Here's how the part is built. I have some questions about the finished solid (model axes, mm). Face numbers are marked on the shaded views. Round coordinates to 2 decimals unless told otherwise and drop trailing zeros. Order: outer loops, then holes, each group sorted by start corner. A loop starts at its lowest first (then second) coordinate and runs counter-clockwise, first axis right, second up. Notation, with made-up numbers: (25.25, 86.25) -> (58.25, 86.25) arc R29 ccw to (58.25, 106.25) -> close; hole circle Ø4 at (82.25, -4). An arc over 180 degrees is marked (long way). One line per item, written item: value.
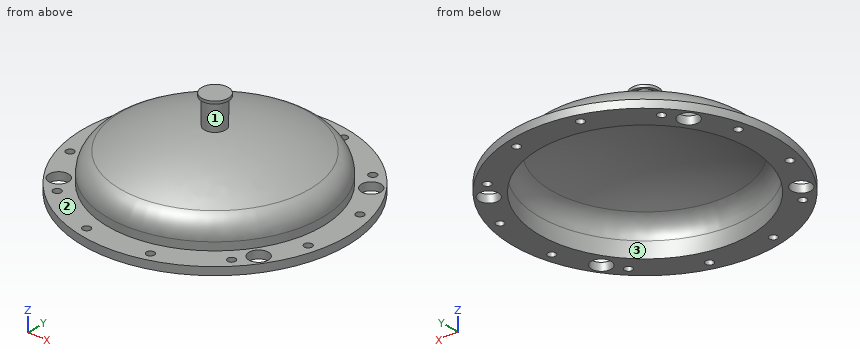
```python
from build123d import *

# Parameters (mm, degrees)
F2_R          = 250
F2_R_2        = 200
F3_DEPTH      = 10
F3_DEPTH_BACK = 5
F4_R          = 7.5
F5_DEPTH      = 15
F7_R          = 20
F9_R          = 25.25
F10_DEPTH     = 5
F11_R         = 18.5
F12_DEPTH     = 20


with BuildPart() as f1:
    # F0 (on Front) → F1 (revolve)
    with BuildSketch(Plane.XZ):
        with BuildLine():
            Line((200, 20), (200, 0))
            Line((200, 0), (203, 0))
            Line((203, 0), (203, 20))
            ThreePointArc((203, 20), (196.5493669363, 42.6526770285), (179.1328476019, 58.5088839444))
            ThreePointArc((179.1328476019, 58.5088839444), (92.0009441475, 89.9153591058), (0, 100.6000003082))
            Line((0, 100.6000003082), (0, 97.6))
            ThreePointArc((0, 97.6), (91.3153782925, 86.994742746), (177.7979977692, 55.8222176227))
            ThreePointArc((177.7979977692, 55.8222176227), (193.9994111035, 41.072257701), (200, 20))
        make_face()
    revolve(axis=Axis((0, 0, 99.1000001541), (0, 0, 1)))

    # F2 (on face) → F3 (join, two sides)
    with BuildSketch(Plane(origin=(0, 0, 0), x_dir=(1, 0, 0), z_dir=(0, 0, -1))) as f3_sk:
        Circle(F2_R)
        Circle(F2_R_2, mode=Mode.SUBTRACT)
    extrude(amount=F3_DEPTH)
    extrude(f3_sk.sketch, amount=-F3_DEPTH_BACK)

    # F4 (on face) → F5 (cut, through all)
    with BuildSketch(Plane.XY.offset(5)):
        with Locations((222.8771156759, 58.8813327608)):
            Circle(F4_R)
        with Locations((163.5765777171, 162.4312878175)):
            Circle(F4_R)
        with Locations((60.4458278584, 222.457910478)):
            Circle(F4_R)
        with Locations((-58.8813327608, 222.8771156759)):
            Circle(F4_R)
        with Locations((-162.4312878175, 163.5765777171)):
            Circle(F4_R)
        with Locations((-222.457910478, 60.4458278584)):
            Circle(F4_R)
        with Locations((-222.8771156759, -58.8813327608)):
            Circle(F4_R)
        with Locations((-163.5765777171, -162.4312878175)):
            Circle(F4_R)
        with Locations((-60.4458278584, -222.457910478)):
            Circle(F4_R)
        with Locations((58.8813327608, -222.8771156759)):
            Circle(F4_R)
        with Locations((162.4312878175, -163.5765777171)):
            Circle(F4_R)
        with Locations((222.457910478, -60.4458278584)):
            Circle(F4_R)
    extrude(amount=-F5_DEPTH, mode=Mode.SUBTRACT)

    # F7 (on offset) → F8 (join, up to the next surface of F1)
    with BuildSketch(Plane.XY.offset(150)):
        Circle(F7_R)
    extrude(until=Until.NEXT, dir=(0, 0, -1))

    # F9 (on face) → F10 (join)
    with BuildSketch(Plane.XY.offset(150)):
        Circle(F9_R)
    extrude(amount=F10_DEPTH)

    # F11 (on face) → F12 (cut)
    with BuildSketch(Plane.XY.offset(5)):
        with Locations((186.3570900757, 130.4886392699)):
            Circle(F11_R)
        with Locations((-186.3570900757, 130.4886392699)):
            Circle(F11_R)
        with Locations((-186.3570900757, -130.4886392699)):
            Circle(F11_R)
        with Locations((186.3570900757, -130.4886392699)):
            Circle(F11_R)
    extrude(amount=-F12_DEPTH, mode=Mode.SUBTRACT)


solid = f1.part
```
Q1. If we mould it in two halves opening along X, with no side actions, what happens to the marked faces 1, 2 and 3? For each: pulls with the +X half, pulls with the -X half, needs draft (parallel to the pull), parting line crosses it, or undercut.
Answers:
face 1: parting line crosses it
face 2: needs draft
face 3: undercut
Q2. For P1, Ø12, axis at x = 194, y = 26.5, coming from the +Z side; P2, Ø3, axis at x = -76.5, z = 56.5, coming from the +Y side; P3, Ø1, axis at y = 100, z = 21.5, coming from the -X side, each with a flat end and sliding along its axis, tell me the tip position at first contact or that it passes through.
Answers:
P1: z = 51
P2: y = 168.52
P3: x = -176.91
Q3. I want a section at A-A on z = 131. Write out the boundary of the cut face in (x, y).
Answers:
outline: circle Ø40 at (0, 0)
Q4. I need wall thicknesses on line 1 along X through (y, z) = (58, 2.5); line 2 along Z through (x, y) = (-155, -179); line 3 along Y through (x, z) = (-176.5, -3). Which ranges of each line are inside material? Lowest first, please.
Answers:
line 1: -243.18 to -229.55, -215.37 to -191.41, 191.41 to 215.43, 230.33 to 243.18
line 2: -10 to 5
line 3: -177.05 to -146.14, -114.83 to -94.06, 94.06 to 114.83, 146.14 to 177.05
